Verification items for the finished model (mm, model axes). A direction names the side the tool comes from. Round coordinates to 2 decimals unless told otherwise and drop trailing zeros. Order: outer loops, then holes, each group sorted by start corner. A loop starts at its lowest first (then second) coordinate and runs counter-clockwise, first axis right, second up. Notation, with made-up numbers: (59, 69.5) -> (96, 69.5) arc R19 ccw to (96, 106.5) -> close; hole circle Ø2 at (29.5, -12). An arc over 180 degrees is marked (long way). Put each result on its own line as item: value.
from build123d import *
from OCP.BRepFilletAPI import BRepFilletAPI_MakeChamfer

# Parameters (mm, degrees)
SKETCH1_W           = 60
SKETCH1_H           = 45
BOSS_EXTRUDE1_DEPTH = 30
SKETCH2_W           = 6.5
SKETCH2_H           = 16
CUT_EXTRUDE1_DEPTH  = 20
CHAMFER1_SIZE       = 5
CHAMFER1_SIZE2      = 0.437443318
CHAMFER2_SIZE       = 5
CHAMFER2_SIZE2      = 5.958767963
CUT_EXTRUDE2_DEPTH  = 10
CHAMFER3_SIZE       = 3
CHAMFER3_SIZE2      = 1.5
CUT_EXTRUDE3_REACH  = 82.777
SKETCH6_W           = 28
SKETCH6_H           = 31
CUT_EXTRUDE4_DEPTH  = 1


with BuildPart() as part:
    # Sketch1 → Boss-Extrude1 (new body)
    with BuildSketch(Plane(origin=(0, 0, 0), x_dir=(1, 0, 0), z_dir=(0, 1, 0))):
        with Locations((-30, 22.5)):
            Rectangle(SKETCH1_W, SKETCH1_H)
    extrude(amount=BOSS_EXTRUDE1_DEPTH)

    # Sketch2 → Cut-Extrude1 (cut)
    with BuildSketch(Plane(origin=(0, 0, 0), x_dir=(-1, 0, 0), z_dir=(0, -1, 0))):
        with Locations((47.5, 21)):
            Rectangle(SKETCH2_W, SKETCH2_H)
        with Locations((13, 21)):
            Rectangle(SKETCH2_W, SKETCH2_H)
    extrude(amount=-CUT_EXTRUDE1_DEPTH, mode=Mode.SUBTRACT)

    # Chamfer1: one chamfer whose edges measure the first distance from different faces: ONE call of the kernel's chamfer builder (chamfer() names one face for all edges)
    chamfer1_edges_1 = [part.edges().sort_by_distance(p)[0] for p in [
        (-50.75, 20, -21),
    ]]
    chamfer1_side_1 = [part.faces().sort_by_distance(p)[0] for p in [
        (-50.75, 10, -21),
    ]]
    chamfer1_edges_2 = [part.edges().sort_by_distance(p)[0] for p in [
        (-44.25, 20, -21),
    ]]
    chamfer1_side_2 = [part.faces().sort_by_distance(p)[0] for p in [
        (-44.25, 10, -21),
    ]]
    chamfer1_edges_3 = [part.edges().sort_by_distance(p)[0] for p in [
        (-16.25, 20, -21),
    ]]
    chamfer1_side_3 = [part.faces().sort_by_distance(p)[0] for p in [
        (-16.25, 10, -21),
    ]]
    chamfer1_edges_4 = [part.edges().sort_by_distance(p)[0] for p in [
        (-9.75, 20, -21),
    ]]
    chamfer1_side_4 = [part.faces().sort_by_distance(p)[0] for p in [
        (-9.75, 10, -21),
    ]]
    chamfer1 = BRepFilletAPI_MakeChamfer(part.part.solid().wrapped)
    for e in chamfer1_edges_1:
        chamfer1.Add(CHAMFER1_SIZE, CHAMFER1_SIZE2, e.wrapped, chamfer1_side_1[0].wrapped)  # the first distance lies on this face
    for e in chamfer1_edges_2:
        chamfer1.Add(CHAMFER1_SIZE, CHAMFER1_SIZE2, e.wrapped, chamfer1_side_2[0].wrapped)  # the first distance lies on this face
    for e in chamfer1_edges_3:
        chamfer1.Add(CHAMFER1_SIZE, CHAMFER1_SIZE2, e.wrapped, chamfer1_side_3[0].wrapped)  # the first distance lies on this face
    for e in chamfer1_edges_4:
        chamfer1.Add(CHAMFER1_SIZE, CHAMFER1_SIZE2, e.wrapped, chamfer1_side_4[0].wrapped)  # the first distance lies on this face
    add(Compound.cast(chamfer1.Shape()), mode=Mode.REPLACE)

    # Chamfer2: one chamfer whose edges measure the first distance from different faces: ONE call of the kernel's chamfer builder (chamfer() names one face for all edges)
    chamfer2_edges_1 = [part.edges().sort_by_distance(p)[0] for p in [
        (-47.5, 20, -29),
    ]]
    chamfer2_side_1 = [part.faces().sort_by_distance(p)[0] for p in [
        (-47.5, 9.857394508, -29),
    ]]
    chamfer2_edges_2 = [part.edges().sort_by_distance(p)[0] for p in [
        (-13, 20, -29),
    ]]
    chamfer2_side_2 = [part.faces().sort_by_distance(p)[0] for p in [
        (-13, 9.857394508, -29),
    ]]
    chamfer2_edges_3 = [part.edges().sort_by_distance(p)[0] for p in [
        (-13, 20, -13),
    ]]
    chamfer2_side_3 = [part.faces().sort_by_distance(p)[0] for p in [
        (-13, 9.857394508, -13),
    ]]
    chamfer2_edges_4 = [part.edges().sort_by_distance(p)[0] for p in [
        (-47.5, 20, -13),
    ]]
    chamfer2_side_4 = [part.faces().sort_by_distance(p)[0] for p in [
        (-47.5, 9.857394508, -13),
    ]]
    chamfer2 = BRepFilletAPI_MakeChamfer(part.part.solid().wrapped)
    for e in chamfer2_edges_1:
        chamfer2.Add(CHAMFER2_SIZE, CHAMFER2_SIZE2, e.wrapped, chamfer2_side_1[0].wrapped)  # the first distance lies on this face
    for e in chamfer2_edges_2:
        chamfer2.Add(CHAMFER2_SIZE, CHAMFER2_SIZE2, e.wrapped, chamfer2_side_2[0].wrapped)  # the first distance lies on this face
    for e in chamfer2_edges_3:
        chamfer2.Add(CHAMFER2_SIZE, CHAMFER2_SIZE2, e.wrapped, chamfer2_side_3[0].wrapped)  # the first distance lies on this face
    for e in chamfer2_edges_4:
        chamfer2.Add(CHAMFER2_SIZE, CHAMFER2_SIZE2, e.wrapped, chamfer2_side_4[0].wrapped)  # the first distance lies on this face
    add(Compound.cast(chamfer2.Shape()), mode=Mode.REPLACE)

    # Sketch4 → Cut-Extrude2 (cut)
    with BuildSketch(Plane(origin=(0, 0, -45), x_dir=(-1, 0, 0), z_dir=(0, 0, -1))):
        with BuildLine():
            Line((11.5, 0), (28.3, 0))
            ThreePointArc((28.3, 0), (34.080602383, 6.276082414), (42.61191296, 6.13008847))
            ThreePointArc((42.61191296, 6.13008847), (47.088831578, 7.478397416), (46.230644896, 12.074510224))
            ThreePointArc((46.230644896, 12.074510224), (25.608734298, 15.404376803), (11.5, 0))
        make_face()
    extrude(amount=-CUT_EXTRUDE2_DEPTH, mode=Mode.SUBTRACT)

    # Chamfer3
    chamfer3_edges = [part.edges().sort_by_distance(p)[0] for p in [
        (-50.75, 0, -21),
        (-47.5, 0, -29),
        (-44.25, 0, -21),
        (-47.5, 0, -13),
        (-16.25, 0, -21),
        (-13, 0, -29),
        (-9.75, 0, -21),
        (-13, 0, -13),
    ]]
    chamfer3_side = [part.faces().sort_by_distance(p)[0] for p in [
        (-30.707745267, 0, -21.36919105),
    ]]
    chamfer(chamfer3_edges, length=CHAMFER3_SIZE, length2=CHAMFER3_SIZE2, reference=chamfer3_side[0])

    # Sketch5 → Cut-Extrude3 (cut, up to next)
    with BuildSketch(Plane.ZY.offset(60), mode=Mode.PRIVATE) as cut_extrude3_sk1:
        Polygon((-45, 30), (0, 30), (0, 0), (-6, 0), (-6, 22), (-45, 22), align=None)
    cut_extrude3_tool1 = extrude(cut_extrude3_sk1.sketch, amount=-CUT_EXTRUDE3_REACH, mode=Mode.PRIVATE) & part.part
    add(cut_extrude3_tool1.solids().sort_by_distance((-60, 29.459167, -22.5))[0], mode=Mode.SUBTRACT)

    # Sketch6 → Cut-Extrude4 (cut)
    with BuildSketch(Plane(origin=(0, 0, 0), x_dir=(-1, 0, 0), z_dir=(0, -1, 0))):
        with Locations((30.25, 21.5)):
            Rectangle(SKETCH6_W, SKETCH6_H)
    extrude(amount=-CUT_EXTRUDE4_DEPTH, mode=Mode.SUBTRACT)


solid = part.part
Item 1: Material ranges on L1, parallel to X at y = 3.25, z = -25.5; L2, parallel to X at y = 19.25, z = -21; L3, parallel to Z at x = -33, y = 9, recorded low to high. Write a range as [from, to].
Check sheet entries:
L1: x = [-60, -50.75], [-44.25, -16.25], [-9.75, 0]
L2: x = [-60, -50.38], [-44.62, -15.88], [-10.12, 0]
L3: z = [-35, -6]
Item 2: Section check B-B on y = 2.75. Record the boundary of the cut face in (x, z).
Check sheet entries:
outline: (-60, -45) -> (-29.7, -45) -> (-29.7, -35) -> (-12.39, -35) -> (-12.39, -45) -> (0, -45) -> (0, -6) -> (-60, -6) -> close; hole (-50.75, -29) -> (-44.25, -29) -> (-44.25, -13) -> (-50.75, -13) -> close; hole (-16.25, -29) -> (-9.75, -29) -> (-9.75, -13) -> (-16.25, -13) -> close
Item 3: Tool access check on faces 1 (the flat face through (-30, 11, -6)), 2 (the flat face through (-44.25, 8, -21)), 3 (the cylindrical face through (-33.97, 6.23, -40.07)). Record the directions out of +Z, -Z, +X, -X, +Y, -Y that give a thin tool (end or side, any length) a straight path to the whole face; none if there is none.
Check sheet entries:
face 1: +Z, +X, -X, +Y, -Y
face 2: -Y
face 3: -Z
Item 4: Section check C-C on x = -49.5. Record the boundary of the cut face in (y, z), then the cut area to 3 significant figures.
Check sheet entries:
outline: (0, -45) -> (22, -45) -> (22, -6) -> (0, -6) -> (0, -10) -> (1.5, -13) -> (15, -13) -> (20, -18.96) -> (20, -23.04) -> (15, -29) -> (1.5, -29) -> (0, -32) -> close
area: 563 mm^2
Item 5: Section check A-A on z = -22. Record the boundary of the cut face in (x, y), then the cut area to 3 significant figures.
Check sheet entries:
outline: (-60, 0) -> (-53.75, 0) -> (-50.75, 1.5) -> (-50.75, 15) -> (-50.31, 20) -> (-44.69, 20) -> (-44.25, 15) -> (-44.25, 1.5) -> (-43.25, 1) -> (-17.25, 1) -> (-16.25, 1.5) -> (-16.25, 15) -> (-15.81, 20) -> (-10.19, 20) -> (-9.75, 15) -> (-9.75, 1.5) -> (-6.75, 0) -> (0, 0) -> (0, 22) -> (-60, 22) -> close
area: 1,030 mm^2
Item 6: Gauge pin test, flat ends, axial feed: pin 1 Ø3.5 at (x, z) = (-12.5, -20) entering from -Y; pin 2 Ø0.5 at (x, y) = (-33, 0.5) entering from +Z; pin 3 Ø1.2 at (x, z) = (-46.5, -21.5) entering from -Y. Record the tip position at first contact, or that the pin passes through.
Check sheet entries:
pin 1: stops at y = 19.41
pin 2: stops at z = -37
pin 3: stops at y = 20
Item 7: Section check D-D on y = 8.75. Record the boundary of the cut face in (x, z), then the cut area to 3 significant figures.
Check sheet entries:
outline: (-60, -45) -> (-47.56, -45) -> (-47.56, -35) -> (-15.97, -35) -> (-15.97, -45) -> (0, -45) -> (0, -6) -> (-60, -6) -> close; hole (-50.75, -29) -> (-44.25, -29) -> (-44.25, -13) -> (-50.75, -13) -> close; hole (-16.25, -29) -> (-9.75, -29) -> (-9.75, -13) -> (-16.25, -13) -> close
area: 1,820 mm^2
Item 8: Release check for a two-part mould opening along X. For faces 4 (the cylindrical face through (-47.051, 7.418, -40.07)), 5 (the flat face through (-48, 0, -34)), 6 (the flat face through (-44.423, 16.979, -20.888)) record: +X half, -X half, draft (parallel to the pull), parting line (faces both ways), or undercut.
Check sheet entries:
face 4: undercut
face 5: draft
face 6: undercut
